Read the model definition and answer for the solid it produces. Units are mm, in the model's axes. A direction names the side the tool comes from. Give positions to 0.01 mm unless a question says otherwise; leave off trailing zeros. Loops run counter-clockwise (first coordinate to the right, second up) from the corner with the lowest first, then second, coordinate; pieces in that order, holes last. Notation, with made-up numbers: (-27, 38) - (-21, 38) arc R18 cw to (-21, 71) - close; hole circle Ø8 at (-25, 32.25). An arc over 180 degrees is marked (long way). Put each result on its own line as item: value. Start each with the question number.
1. Given pin 1 Ø7.5 at (x, y) = (125.5, 54) entering from -Z; pin 2 Ø1.9 at (x, z) = (134, 4.5) entering from +Y; pin 3 Ø3 at (y, z) = (38, 5.5) entering from +X, each flat-ended and moving along its own axis, determine where each tip first touches the part or whether it passes through.
2. A cutting plane is placed at B-B, the plane x = 87.5. Determine the outline of the cut face in (y, z), plus the area to 3 significant figures.
3. A cutting plane is placed at C-C, the plane z = -2. Determine the outline of the cut face in (x, y) (3 decimals).
4. For faces 4 (the flat face through (114.25, 36, 4)), 5 (the flat face through (60, 2.75, 4)), 6 (the flat face through (131, 44.75, 5)), determine the directions among +Z, -Z, +X, -X, +Y, -Y from which every point of the face is accessible in a straight line to the end or side of a thin tool.
5. A cutting plane is placed at D-D, the plane y = 49. Determine the outline of the cut face in (x, z).
6. For a pull along Y with two mould halves and no side action, classify faces 1 (the flat face through (60, 40, 6.25)), 2 (the flat face through (19, 40.5, -5)), 3 (the flat face through (126, 56, -5.5)) as released by +Y, released by -Y, zero draft, split by the parting line, or undercut.
7. Consider L1, parallel to Z at x = 15, y = 44.5; L2, parallel to Y at x = 67, z = 2.5; L3, parallel to Z at x = 12, y = 69. Determine where each line is inside the solid, lowest interval first. Write a range as from..to.
8. A cutting plane is placed at A-A, the plane y = 38.75. Determine the outline of the cut face in (x, z).
```python
from build123d import *

# Parameters (mm, degrees)
SKETCH_W        = 141
SKETCH_H        = 73.5
PAD_DEPTH       = 1.75
SKETCH001_W     = 106.75
SKETCH001_H     = 68.25
PAD001_DEPTH    = 5
SKETCH002_W     = 98.75
SKETCH002_H     = 57
POCKET_DEPTH    = 0.5
SKETCH003_W     = 12.5
SKETCH003_H     = 12
PAD002_DEPTH    = 6.35
SKETCH004_R     = 3.5
PAD003_DEPTH    = 14.75
SKETCH005_R     = 4.625
PAD004_DEPTH    = 5.5
SKETCH006_W     = 9
SKETCH006_H     = 20.5
PAD005_DEPTH    = 9.5
SKETCH007_R     = 1.6665
POCKET001_DEPTH = 11.251


with BuildPart() as part:
    # Sketch → Pad (new body)
    with BuildSketch(Plane.XY):
        with Locations((70.5, 36.75)):
            Rectangle(SKETCH_W, SKETCH_H)
    extrude(amount=PAD_DEPTH)

    # Sketch001 (on Face6 of Pad) → Pad001 (join)
    with BuildSketch(Plane.XY.offset(1.75)):
        with Locations((60.875, 36.875)):
            Rectangle(SKETCH001_W, SKETCH001_H)
    extrude(amount=PAD001_DEPTH)

    # Sketch002 (on Face11 of Pad001) → Pocket (cut)
    with BuildSketch(Plane.XY.offset(6.75)):
        with Locations((60.875, 39.25)):
            Rectangle(SKETCH002_W, SKETCH002_H)
    extrude(amount=-POCKET_DEPTH, mode=Mode.SUBTRACT)

    # Sketch003 (on Face5 of Pocket) → Pad002 (join)
    with BuildSketch(Plane.XY.offset(1.75)):
        with Locations((131.5, 38.75)):
            Rectangle(SKETCH003_W, SKETCH003_H)
    extrude(amount=PAD002_DEPTH)

    # Sketch004 (on Face16 of Pad002) → Pad003 (join)
    with BuildSketch(Plane.XY.offset(8.1)):
        with Locations((131.5, 38.75)):
            Circle(SKETCH004_R)
    extrude(amount=PAD003_DEPTH)

    # Sketch005 (on Face4 of Pad003) → Pad004 (join)
    with BuildSketch(Plane(origin=(0, 0, 0), x_dir=(1, 0, 0), z_dir=(0, 0, -1))):
        with Locations((125.725, -55.875)):
            Circle(SKETCH005_R)
    extrude(amount=PAD004_DEPTH)

    # Sketch006 (on Face4 of Pad004) → Pad005 (join)
    with BuildSketch(Plane(origin=(0, 0, 0), x_dir=(1, 0, 0), z_dir=(0, 0, -1))):
        with Locations((19.5, -30.25)):
            Rectangle(SKETCH006_W, SKETCH006_H)
    extrude(amount=PAD005_DEPTH)

    # Sketch007 (on Face5 of Pad005) → Pocket001 (cut, through all)
    with BuildSketch(Plane.XY.offset(1.75)):
        with Locations((3.1665, 3.6665)):
            Circle(SKETCH007_R)
        with Locations((3.1665, 69.8335)):
            Circle(SKETCH007_R)
        with Locations((118.2835, 3.6665)):
            Circle(SKETCH007_R)
        with Locations((118.2835, 69.8335)):
            Circle(SKETCH007_R)
    extrude(amount=-POCKET001_DEPTH, mode=Mode.SUBTRACT)


solid = part.part
```
Return value:
1. pin 1: stops at z = -5.5
1. pin 2: stops at y = 44.75
1. pin 3: stops at x = 137.75
2. outline: (0, 0) - (73.5, 0) - (73.5, 1.75) - (71, 1.75) - (71, 6.75) - (67.75, 6.75) - (67.75, 6.25) - (10.75, 6.25) - (10.75, 6.75) - (2.75, 6.75) - (2.75, 1.75) - (0, 1.75) - close
2. area: 441 mm2
3. outline: (15, 20) - (24, 20) - (24, 40.5) - (15, 40.5) - close; circle Ø9.25 at (125.725, 55.875)
4. face 4: +Z, +Y, -Y
4. face 5: +Z, +X, -X, -Y
4. face 6: +Z, +X, +Y
5. outline: (0, 0) - (141, 0) - (141, 1.75) - (114.25, 1.75) - (114.25, 6.75) - (110.25, 6.75) - (110.25, 6.25) - (11.5, 6.25) - (11.5, 6.75) - (7.5, 6.75) - (7.5, 1.75) - (0, 1.75) - close
6. face 1: undercut
6. face 2: released by +Y
6. face 3: zero draft
7. L1: z = 0..6.25
7. L2: y = 2.75..71
7. L3: z = 0..6.75
8. outline: (0, 0) - (15, 0) - (15, -9.5) - (24, -9.5) - (24, 0) - (141, 0) - (141, 1.75) - (137.75, 1.75) - (137.75, 8.1) - (135, 8.1) - (135, 22.85) - (128, 22.85) - (128, 8.1) - (125.25, 8.1) - (125.25, 1.75) - (114.25, 1.75) - (114.25, 6.75) - (110.25, 6.75) - (110.25, 6.25) - (11.5, 6.25) - (11.5, 6.75) - (7.5, 6.75) - (7.5, 1.75) - (0, 1.75) - close
